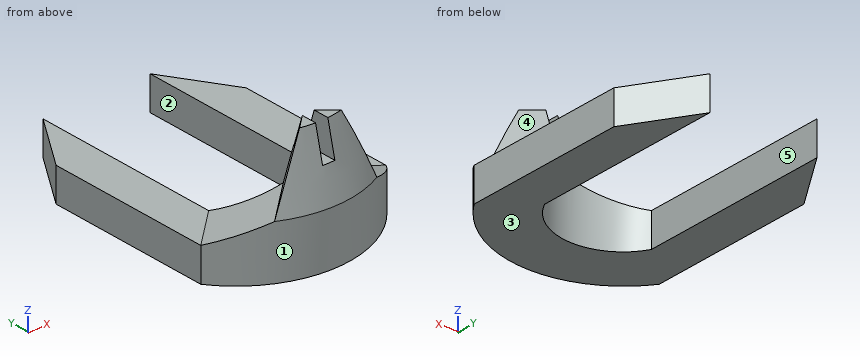
from build123d import *

# Parameters (mm, degrees)
F1_DEPTH    = 40
F2_DEPTH    = 25
F3_DEPTH    = 25
F4_SIZE2    = 41.212151
F4_SIZE     = 14.99999
F4_2_SIZE2  = 41.212151
F4_2_SIZE   = 14.99999
F5_DEPTH    = 25
F8_DEPTH    = 25
F9_T1_DEPTH = 305.3611948779
F9_T3_DEPTH = 305.3964050976
F9_T6_ANGLE = 198.1358920289
F9_T8_ANGLE = 199.0272584804


# Not quite as in the source:
# - a fillet or chamfer that OpenCascade refuses, or shapes differently, is made with other operations: its cross-section is extruded or revolved along the edge and cut away or added
# - a fillet or chamfer is up to 0.001 mm smaller than in the source, because OpenCascade refuses the exact size
# - ends of sketch curves that miss each other by under 0.0002 mm in the source are joined
# - a feature of the source that left no trace in its solid (it failed there, or was rolled back) is left out


with BuildPart() as f1:
    # F0 (on Top) → F1 (new body)
    with BuildSketch(Plane.XY):
        with BuildLine():
            Line((-40, -36.0045238119), (-70, -63.6819600925))
            ThreePointArc((-70, -63.6819600925), (0.5336536193, -99.3066602871), (70, -61.643119862))
            Line((70, -61.643119862), (40, -35.7918441296))
            ThreePointArc((40, -35.7918441296), (0.0635323292, -59.7960301521), (-40, -36.0045238119))
        make_face()
    extrude(amount=F1_DEPTH)

    # F0 (on Top) → F2 (join)
    with BuildSketch(Plane.XY):
        Polygon((-40, 105.9954761881), (-70, 60.3440771007), (-70, -63.6819600925), (-40, -36.0045238119), align=None)
    extrude(amount=F2_DEPTH)

    # F0 (on Top) → F3 (join)
    with BuildSketch(Plane.XY):
        Polygon((40, -35.7918441296), (70, -61.643119862), (70, 58.0248532689), (40, 105.9954761881), align=None)
    extrude(amount=F3_DEPTH)

    # F4 (size 15 and 41.2121612918 in the source; OpenCascade refuses exactly that, so slightly less here)
    f4_edges = [f1.edges().sort_by_distance(p)[0] for p in [
        (55, -48.717482, 40),
    ]]
    f4_side = f1.faces().sort_by_distance((55, -48.717482, 32.5))[0]
    chamfer(f4_edges, length=F4_SIZE, length2=F4_SIZE2, reference=f4_side)

    # F4#2 (size 15 and 41.2121612918 in the source; OpenCascade refuses exactly that, so slightly less here)
    f4_2_edges = [f1.edges().sort_by_distance(p)[0] for p in [
        (-55, -49.843242, 40),
    ]]
    f4_2_side = f1.faces().sort_by_distance((-55, -49.843242, 32.5))[0]
    chamfer(f4_2_edges, length=F4_2_SIZE, length2=F4_2_SIZE2, reference=f4_2_side)

    # F5 (add): a face of the model
    f5_faces = [f1.faces().sort_by_distance(p)[0] for p in [
        (0.2353529627, -82.8231732058, 40),
    ]]
    extrude(f5_faces, amount=F5_DEPTH)

    # F6 (on face) → F8 (join)
    with BuildSketch(Plane.XY.offset(65)):
        with BuildLine():
            Line((-4.7475561509, -99.219810589), (-4.7475561509, -59.5533930445))
            Line((-4.7475561509, -59.5533930445), (-38.3453534122, -90.5500754708))
            ThreePointArc((-38.3453534122, -90.5500754708), (-21.992530831, -96.6136201427), (-4.7475561509, -99.219810589))
        make_face()
        with BuildLine():
            Line((39.117860909, -89.4339641513), (4.4621424554, -59.5708130363))
            Line((4.4621424554, -59.5708130363), (4.4621283286, -99.1587323277))
            ThreePointArc((4.4621283286, -99.1587323277), (22.3094657758, -96.1475649652), (39.117860909, -89.4339641513))
        make_face()
    extrude(amount=F8_DEPTH)

    # F9: chamfer of 12 x 49.9835972411 on 4 edges, made by hand

    # F9_s2 → F9_t1 (cut)
    with BuildSketch(Plane(origin=(63.1741452332, 58.2832529798, 0), x_dir=(0, 0, 1), z_dir=(-0.73498516, -0.6780831915, 0))):
        Polygon((40.0164027589, -40.5516220902), (90, -52.5516220902), (90, -40.5516220902), align=None)
    extrude(amount=F9_T1_DEPTH, mode=Mode.SUBTRACT)

    # F9_s4 → F9_t3 (cut)
    with BuildSketch(Plane(origin=(165.0227982776, -142.2016620137, 0), x_dir=(0, 0, 1), z_dir=(-0.7575447308, 0.6527832572, 0))):
        Polygon((90, -54.2147436385), (40.0164027589, -42.2147436385), (90, -42.2147436385), align=None)
    extrude(amount=F9_T3_DEPTH, mode=Mode.SUBTRACT)

    # F9_s5 → F9_t6 (revolve, cut)
    with BuildSketch(Plane(origin=(-5.284270337, -12.1314567966, 0), x_dir=(0, 0, 1), z_dir=(0.3993440485, 0.9168011404, 0))):
        Polygon((90, -68.1975743243), (40.0164027589, -80.1975743243), (90, -80.1975743243), align=None)
    revolve(axis=Axis((-0.7068547451, -14.1253064914, 90), (0, 0, 1)), revolution_arc=F9_T6_ANGLE, mode=Mode.SUBTRACT)

    # F9_s7 → F9_t8 (revolve, cut)
    with BuildSketch(Plane(origin=(1.4990811594, -13.8871820878, 0), x_dir=(0, 0, 1), z_dir=(-0.1073236217, 0.9942241398, 0))):
        Polygon((40.0164027589, -87.4091372686), (90, -75.4091372686), (90, -87.4091372686), align=None)
    revolve(axis=Axis((-0.7068547451, -14.1253064914, 90), (0, 0, 1)), revolution_arc=F9_T8_ANGLE, mode=Mode.SUBTRACT)


solid = f1.part
Geometry check sheet. Reference: the model listing, model coordinates, mm. Face numbers are marked on the shaded views. A direction names the side the tool comes from. Give positions to 0.01 mm unless a question says otherwise; leave off trailing zeros. Order: outer loops, then holes, each group sorted by start corner. A loop starts at its lowest first (then second) coordinate and runs counter-clockwise, first axis right, second up.
1. Sectioned sample at D-D (y = 89). Record the boundary of the cut face in (x, z), then the cut area to 3 significant figures.
Completed:
outline: (-51.17, 0) - (-40, 0) - (-40, 25) - (-51.17, 25) - close; (40, 0) - (50.63, 0) - (50.63, 25) - (40, 25) - close
area: 545 mm2
2. Sectioned sample at C-C (z = 83). Record the boundary of the cut face in (x, y), then the cut area to 3 significant figures.
Completed:
outline: (-18.99, -86.73) arc R74.87 ccw to (-4.75, -88.89) - (-4.75, -73.59) - close; (4.46, -88.82) arc R74.87 ccw to (19.56, -86.2) - (4.46, -73.19) - close
area: 234 mm2
3. Access from +Z, -Z, +X, -X, +Y, -Y to the whole of each face (thin tool, end or side, straight path). Record for the marked faces 4 and 5.
Completed:
face 4: +Z, +X, +Y
face 5: +Z, -Z, +Y
4. Depth check by flat-ended pin: pin 1 (12 mm diameter, centred on x = 22, z = 68, fed in from +Y); pin 2 (5 mm diameter, centred on y = -61, z = 46, fed in from +X); pin 3 (15 mm diameter, centred on x = 55.5, y = 60.5, fed in from +Z). Enter the tip coordinate at first touch or a pass-through.
Completed:
pin 1: stops at y = -78.04
pin 2: stops at x = 6.96
pin 3: stops at z = 25
5. Draft check along X on the marked faces 1, 2 and 3. Enter one of: pulls with the +X half, pulls with the -X half, needs draft (parallel to the pull), parting line crosses it, or undercut.
Completed:
face 1: parting line crosses it
face 2: undercut
face 3: needs draft
6. Sectioned sample at A-A (y = -29.5). Record the boundary of the cut face in (x, z), then the cut area to 3 significant figures.
Completed:
outline: (-70, 0) - (-40, 0) - (-40, 25) - (-70, 25) - close; (40, 0) - (70, 0) - (70, 25) - (40, 25) - close
area: 1,500 mm2
7. Sectioned sample at B-B (z = 9). Record the boundary of the cut face in (x, y).
Completed:
outline: (-70, -63.68) arc R85.19 ccw to (70, -61.64) - (70, 58.02) - (40, 106) - (40, -35.79) arc R45.42 cw to (-40, -36) - (-40, 106) - (-70, 60.34) - close
8. Scan lines: line 1 (X direction, y = 30, z = 8.5); line 2 (Z direction, x = -55, y = 83); line 3 (Z direction, x = 0, y = -73). Record each from-to range of solid material in increasing order.
Completed:
line 1: x = -70 to -40, 40 to 70
line 2: z = 0 to 25
line 3: z = 0 to 65
